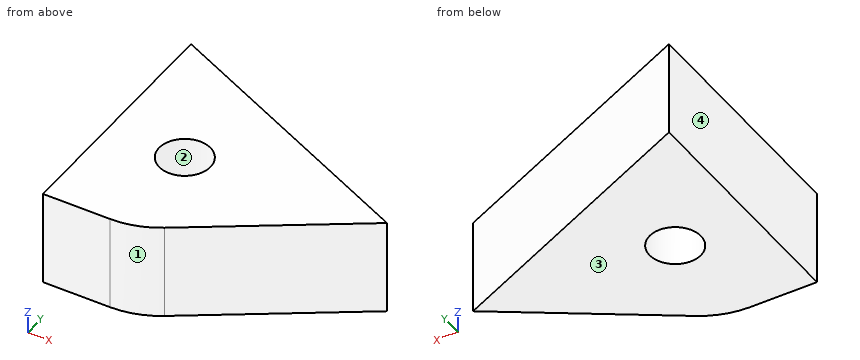
from build123d import *

# Parameters (mm, degrees)
F1_DEPTH = 39.624
F2_R     = 34.885531
F3_R     = 10.6553
F4_DEPTH = 91.186


with BuildPart() as f1:
    # F0 (on Top) → F1 (new body)
    with BuildSketch(Plane.XY):
        Polygon((0, 100.89088), (0, 0), (38.1762, 0), (112.777971, 48.952073), align=None)
    extrude(amount=F1_DEPTH)

    # F2
    f2_edges = [f1.edges().sort_by_distance(p)[0] for p in [
        (38.1762, 0, 19.812),
    ]]
    fillet(f2_edges, radius=F2_R)

    # F3 (on Top) → F4 (cut)
    with BuildSketch(Plane.XY):
        with Locations((31.988665, 44.031467)):
            Circle(F3_R)
    extrude(amount=F4_DEPTH, mode=Mode.SUBTRACT)


solid = f1.part
Input: part model. Units: mm. Frame: model coordinates. Face numbers are marked on the shaded views. Give positions to 0.01 mm unless a question says otherwise; leave off trailing zeros. Write each loop counter-clockwise with the first axis right and the second up, starting at its lowest first coordinate (ties: lowest second). Pieces come first, ordered by that corner, then holes.
Q1. Section B-B, the plane x = 45. Output: boundary loops of the cut face in (y, z), plus the area to 3 significant figures.
Q2. First-contact query: P1, Ø2, axis at x = 67, z = 22, coming from the -Y side; P2, Ø3, axis at x = 41.5, z = 27.5, coming from the +Y side. Flat tips, straight axial feed; report the tip coordinate or a pass-through.
Q3. Section A-A, the plane z = 33.5. Output: boundary loops of the cut face in (x, y).
Q4. Pull-direction query (X, two-part tool) for the marked faces 1, 2, 3 and 4; classes: pulls with the +X half, pulls with the -X half, needs draft (parallel to the pull), parting line crosses it, or undercut.
Q5. Material intervals for probe 1 along Y at (x, z) = (35.5, 16.5); probe 2 along X at (y, z) = (38, 35.5); probe 3 along Y at (x, z) = (29, 24), sorted ascending.
Q6. Section C-C, the plane y = 9.5. Output: boundary loops of the cut face in (x, z).
Filled in:
1. outline: (4.56, 0) - (80.17, 0) - (80.17, 39.62) - (4.56, 39.62) - close
1. area: 3,000 mm2
2. P1: stops at y = 18.26
2. P2: stops at y = 82.47
3. outline: (0, 0) - (27.75, 0) arc R34.89 ccw to (46.89, 5.72) - (112.78, 48.95) - (0, 100.89) - close; hole circle Ø21.31 at (31.99, 44.03)
4. face 1: pulls with the +X half
4. face 2: undercut
4. face 3: needs draft
4. face 4: pulls with the -X half
5. probe 1: y = 0.87 to 33.97, 54.09 to 84.54
5. probe 2: x = 0 to 23.2, 40.77 to 96.09
5. probe 3: y = 0.02 to 33.8, 54.26 to 87.54
6. outline: (0, 0) - (52.65, 0) - (52.65, 39.62) - (0, 39.62) - close
